```python
from build123d import *

# Parameters (mm, degrees)
SKETCH_1_W          = 1960
SKETCH_1_H          = 200
EXTRUDE_1447_DEPTH  = 16
SKETCH_2_W          = 1960
SKETCH_2_H          = 16
EXTRUDE_1_DEPTH     = 104
CUT_EXTRUDE_1_DEPTH = 1008.372820757


with BuildPart() as part:
    # 草图1 → Extrude 1447 (new body)
    with BuildSketch(Plane.XY):
        with Locations((0, 100)):
            Rectangle(SKETCH_1_W, SKETCH_1_H)
    extrude(amount=EXTRUDE_1447_DEPTH)

    # 草图2 → 凸台-拉伸1 (add)
    with BuildSketch(Plane.XY.offset(16)):
        with Locations((0, 192)):
            Rectangle(SKETCH_2_W, SKETCH_2_H)
    extrude(amount=EXTRUDE_1_DEPTH)

    # 草图3 → 切除-拉伸1 (cut, through all)
    with BuildSketch(Plane(origin=(0, 200, 0), x_dir=(-1, 0, 0), z_dir=(0, 1, 0))):
        Polygon((-980, 100), (-830, 120), (-980, 120), align=None)
        Polygon((980, 100), (830, 120), (980, 120), align=None)
    extrude(amount=-CUT_EXTRUDE_1_DEPTH, mode=Mode.SUBTRACT)


solid = part.part
```
Model file for the job. Use its own axes, mm. A direction names the side the tool comes from. Round coordinates to 2 decimals unless told otherwise and drop trailing zeros. Order: outer loops, then holes, each group sorted by start corner. A loop starts at its lowest first (then second) coordinate and runs counter-clockwise, first axis right, second up. Notation, with made-up numbers: (14.25, 64.25) -> (66.25, 64.25) arc R22 cw to (66.25, 71.25) -> close; hole circle Ø1 at (49.25, 86). An arc over 180 degrees is marked (long way). Use one line per item in the form item = value.
Item 1: Tool access for faces 1 (the face through (-980, 129, 13)), 2 (the face through (-14, 184, 67)): list every direction of +Z, -Z, +X, -X, +Y, -Y with a clear straight run to the whole face (end or side of a thin tool).
Returned:
face_1 = +Z, -Z, -X, +Y, -Y
face_2 = +Z, +X, -X, -Y
Item 2: Cut at A-A, the plane x = -770. Write the cut outline in (y, z).
Returned:
outline = (0, 0) -> (200, 0) -> (200, 120) -> (184, 120) -> (184, 16) -> (0, 16) -> close
Item 3: Drill centre lines: line 1 (Y direction, x = -398, z = 45); line 2 (Z direction, x = -727.5, y = 146.5). Where is each one in solid material? Low to high.
Returned:
line_1 = 184 to 200
line_2 = 0 to 16
Item 4: Cut at B-B, the plane z = 32.5. Write the cut outline in (x, y).
Returned:
outline = (-980, 184) -> (980, 184) -> (980, 200) -> (-980, 200) -> close
Item 5: Cut at C-C, the plane y = 109. Write the cut outline in (x, z), and give its area (3 significant figures).
Returned:
outline = (-980, 0) -> (980, 0) -> (980, 16) -> (-980, 16) -> close
area = 31,400 mm^2
Item 6: Flat gauge pins, fed straight in: pin 1 Ø6 at (x, z) = (688.5, 71.5) entering from -Y; pin 2 Ø12 at (x, y) = (-188, 105) entering from +Z. Where does each tip first touch, or does it go through?
Returned:
pin_1 = 184
pin_2 = 16
